Geometry check sheet. Reference: drawing and pictorial views, mm from the part's lowest x, y, z. A direction names the side the tool comes from. Give positions to 0.01 mm unless a question says otherwise; leave off trailing zeros. Loops run counter-clockwise (first coordinate to the right, second up) from the corner with the lowest first, then second, coordinate; pieces in that order, holes last. Notation, with made-up numbers: (66.25, -9) -> (91.25, -9) arc R20 cw to (91.25, 13) -> close; hole circle Ø4 at (72.25, -24.75). An arc over 180 degrees is marked (long way). Write each question's results on one line, items separated by ' | '. Start each with the question number.
1. Cross-section at D-D on y = 8.5. Record the boundary of the cut face in (x, z), and give its area (3 significant figures).
2. Tool access check on the marked faces 4, 5 and 6. Record the directions out of +Z, -Z, +X, -X, +Y, -Y that give a thin tool (end or side, any length) a straight path to the whole face; none if there is none.
3. Cross-section at A-A on y = 40. Record the boundary of the cut face in (x, z), and give its area (3 significant figures).
4. Cross-section at B-B on z = 18.5. Record the boundary of the cut face in (x, y).
5. Mould release check, pull along Y, two halves, no side actions. Record for the marked faces 1, 2 and 3: +Y half, -Y half, draft (parallel to the pull), parting line (faces both ways), or undercut.
6. Gauge pin test, flat ends, axial feed: pin 1 Ø4 at (y, z) = (35.5, 3) entering from +X; pin 2 Ø5 at (y, z) = (31.5, 7) entering from -X; pin 3 Ø8 at (x, y) = (40, 72.5) entering from +Z; pin 4 Ø5 at (x, y) = (7.5, 40) entering from +Z. Record the tip position at first contact, or that the pin passes through.
7. Cross-section at C-C on x = 7.5. Record the boundary of the cut face in (y, z), and give its area (3 significant figures).
8. Material ranges on L1, parallel to Y at x = 40, z = 13.1; L2, parallel to Y at x = 40, z = 15.75; L3, parallel to Z at x = 63, y = 10, recorded low to high. Write a range as from..to.
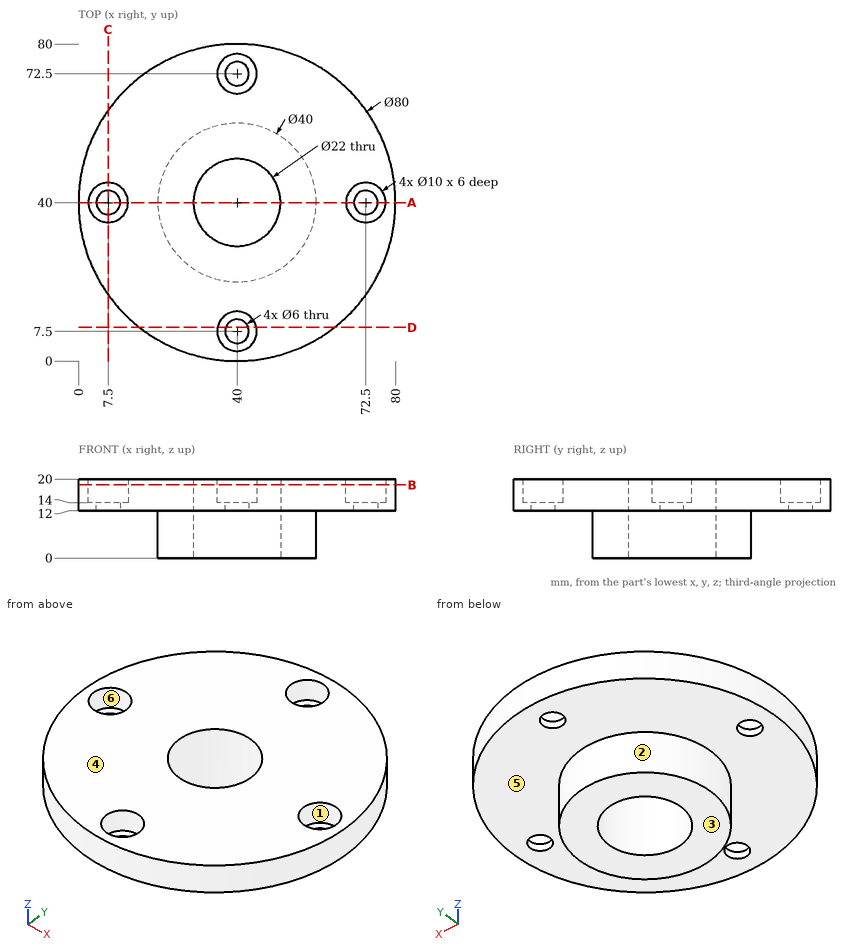
Geometry says:
1) outline: (15.35, 12) -> (37.17, 12) -> (37.17, 14) -> (35.1, 14) -> (35.1, 20) -> (15.35, 20) -> close; (42.83, 12) -> (64.65, 12) -> (64.65, 20) -> (44.9, 20) -> (44.9, 14) -> (42.83, 14) -> close | area: 324 mm^2
2) face 4: +Z, +X, -X, +Y, -Y | face 5: -Z | face 6: +Z
3) outline: (0, 12) -> (4.5, 12) -> (4.5, 14) -> (2.5, 14) -> (2.5, 20) -> (0, 20) -> close; (10.5, 12) -> (20, 12) -> (20, 0) -> (29, 0) -> (29, 20) -> (12.5, 20) -> (12.5, 14) -> (10.5, 14) -> close; (51, 0) -> (60, 0) -> (60, 12) -> (69.5, 12) -> (69.5, 14) -> (67.5, 14) -> (67.5, 20) -> (51, 20) -> close; (75.5, 12) -> (80, 12) -> (80, 20) -> (77.5, 20) -> (77.5, 14) -> (75.5, 14) -> close | area: 536 mm^2
4) outline: circle Ø80 at (40, 40); hole circle Ø10 at (7.5, 40); hole circle Ø22 at (40, 40); hole circle Ø10 at (40, 7.5); hole circle Ø10 at (40, 72.5); hole circle Ø10 at (72.5, 40)
5) face 1: undercut | face 2: parting line | face 3: draft
6) pin 1: x = 59.84 | pin 2: x = 20.92 | pin 3: z = 14 | pin 4: through
7) outline: (16.68, 12) -> (37, 12) -> (37, 14) -> (35, 14) -> (35, 20) -> (16.68, 20) -> close; (43, 12) -> (63.32, 12) -> (63.32, 20) -> (45, 20) -> (45, 14) -> (43, 14) -> close | area: 301 mm^2
8) L1: 0..4.5, 10.5..29, 51..69.5, 75.5..80 | L2: 0..2.5, 12.5..29, 51..67.5, 77.5..80 | L3: 12..20
